Autodesk Inventor part; units mm, degrees
ref_plane "YZ Plane" through (0, 0, 0) normal (1, 0, 0) x (0, 1, 0)
ref_plane "XZ Plane" through (0, 0, 0) normal (0, 1, 0) x (-1, 0, 0)
ref_plane "XY Plane" through (0, 0, 0) normal (0, 0, 1) x (1, 0, 0)
sketch "Sketch1" plane through (0, 0, 0) normal (0, 0, 1) x (1, 0, 0)
  line L0 (-7.5, 73) -> (7.5, 73)
  line L1 (7.5, 73) -> (7.5, 70)
  line L2 (-7.5, 70) -> (-7.5, 73)
  line L3 (-40.4145, 70) -> (-7.5, 70)
  line L4 (7.5, 70) -> (40.4145, 70)
  line L5 (-66.9699, 30.0048) -> (-59.4699, 42.9952)
  line L6 (-59.4699, 42.9952) -> (-56.8718, 41.4952)
  line L7 (-64.3718, 28.5048) -> (-66.9699, 30.0048)
  line L8 (-59.4699, -42.9952) -> (-66.9699, -30.0048)
  line L9 (-66.9699, -30.0048) -> (-64.3718, -28.5048)
  line L10 (-56.8718, -41.4952) -> (-59.4699, -42.9952)
  line L11 (7.5, -73) -> (-7.5, -73)
  line L12 (-7.5, -73) -> (-7.5, -70)
  line L13 (7.5, -70) -> (7.5, -73)
  line L14 (66.9699, -30.0048) -> (59.4699, -42.9952)
  line L15 (59.4699, -42.9952) -> (56.8718, -41.4952)
  line L16 (64.3718, -28.5048) -> (66.9699, -30.0048)
  line L17 (59.4699, 42.9952) -> (66.9699, 30.0048)
  line L18 (66.9699, 30.0048) -> (64.3718, 28.5048)
  line L19 (56.8718, 41.4952) -> (59.4699, 42.9952)
  line L20 (-80.829, 0) -> (-64.3718, 28.5048)
  line L21 (-56.8718, 41.4952) -> (-40.4145, 70)
  line L22 (40.4145, 70) -> (56.8718, 41.4952)
  line L23 (64.3718, 28.5048) -> (80.829, 0)
  line L24 (80.829, 0) -> (64.3718, -28.5048)
  line L25 (56.8718, -41.4952) -> (40.4145, -70)
  line L26 (40.4145, -70) -> (7.5, -70)
  line L27 (-7.5, -70) -> (-40.4145, -70)
  line L28 (-40.4145, -70) -> (-56.8718, -41.4952)
  line L29 (-64.3718, -28.5048) -> (-80.829, 0)
  circle A0 centre (-18.5, 18.5) radius 1.6
  circle A1 centre (18.5, 18.5) radius 1.6
  circle A2 centre (18.5, -18.5) radius 1.6
  circle A3 centre (-18.5, -18.5) radius 1.6
  point P0 (0, 0)
  point P1 (0, 0)
  point P2 (0, 73)
  point P3 (-63.2199, 36.5)
  point P4 (-63.2199, -36.5)
  point P5 (0, -73)
  point P6 (63.2199, -36.5)
  point P7 (63.2199, 36.5)
  dimension "d1" = 3
  dimension "d3" = 15
  dimension "d6" = 360
  dimension "d8" = 140
  dimension "d9" = 146
  dimension "d12" = 3.2
  dimension "d13" = 3.2
  dimension "d14" = 3.2
  dimension "d15" = 3.2
  dimension "d16" = 37
  dimension "d17" = 37
  dimension "d18" = 18.5
  dimension "d19" = 18.5
extrude "Extrusion2" add sketch "Sketch1" along normal blind 3
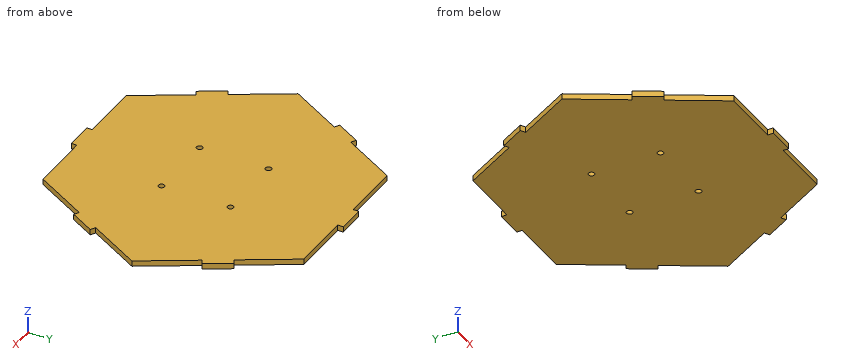
Geometry: final body of the model. Coordinates: model frame, mm. Round coordinates to 2 decimals unless told otherwise and drop trailing zeros. Loops run counter-clockwise (first coordinate to the right, second up) from the corner with the lowest first, then second, coordinate; pieces in that order, holes last.
Item 1: Section B-B, the plane y = 9. Output: boundary loops of the cut face in (x, z), plus the area to 3 significant figures.
Checked values:
outline: (-75.63, 0) - (75.63, 0) - (75.63, 3) - (-75.63, 3) - close
area: 454 mm2
Item 2: Section A-A, the plane z = 2.5. State how many separate pieces and enclosed holes the cut face has, plus the area to 3 significant figures.
Checked values:
separate pieces: 1
enclosed holes: 4
area: 17,200 mm2
Item 3: Contact query for flat-ended pins moving along their axis: P1, Ø1.5, axis at y = -12, z = 0.5, coming from the -X side; P2, Ø0.9, axis at x = -21.5, z = 2, coming from the +Y side; P3, Ø5, axis at x = 18.5, y = 18.5, coming from the +Z side; P4, Ø1.5, axis at x = 31.5, z = 1, coming from the -Y side. Output: stop coordinate, or through.
Checked values:
P1: stops at x = -74.33
P2: stops at y = 70
P3: stops at z = 3
P4: stops at y = -70
Item 4: Line query: L1, parallel to Y at x = 18.5, z = 2.1; L2, parallel to X at y = 19, z = 1.3; L3, parallel to Y at x = 11, z = 0.6. Output: solid intervals per line, ascending.
Checked values:
L1: y = -70 to -20.1, -16.9 to 16.9, 20.1 to 70
L2: x = -69.86 to -20.02, -16.98 to 16.98, 20.02 to 69.86
L3: y = -70 to 70
